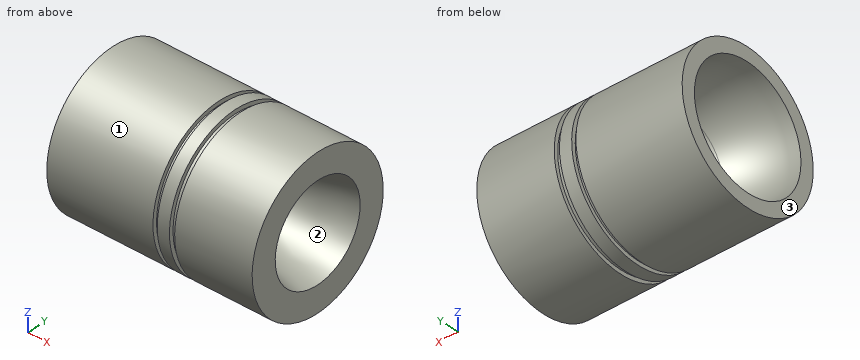
from build123d import *


with BuildPart() as part:
    # Sketch1 → Revolve1 (revolve)
    with BuildSketch(Plane.XY, mode=Mode.PRIVATE) as revolve1_sk:
        with BuildLine():
            Line((43.421005762, 29.901440031), (63.302799643, 18.422680981))
            ThreePointArc((63.302799643, 18.422680981), (68.543849717, 16.213738545), (74.168, 15.367))
            ThreePointArc((74.168, 15.367), (75.003256616, 15.406217174), (75.824358548, 15.564277983))
            Line((75.824358548, 15.564277983), (140.97, 33.02))
            Line((140.97, 33.02), (140.97, 50.927))
            Line((140.97, 50.927), (87.788503876, 50.927))
            Line((87.788503876, 50.927), (87.788503876, 48.180233369))
            Line((87.788503876, 48.180233369), (84.218492297, 48.180233369))
            Line((84.218492297, 48.180233369), (84.218492297, 50.927))
            Line((84.218492297, 50.927), (75.824358548, 50.927))
            Line((75.824358548, 50.927), (75.824358548, 48.180233369))
            Line((75.824358548, 48.180233369), (72.892938323, 48.180233369))
            Line((72.892938323, 48.180233369), (72.892938323, 50.927))
            Line((72.892938323, 50.927), (0, 50.927))
            Line((0, 50.927), (0, 41.402))
            ThreePointArc((0, 41.402), (22.475975666, 38.541805218), (43.421005762, 29.901440031))
        make_face()
    revolve(revolve1_sk.sketch.rotate(Axis((0, 0, 0), (1, 0, 0)), 90), axis=Axis((0, 0, 0), (1, 0, 0)))


solid = part.part
Work out the finished part from the listing and answer in its coordinate system (mm). Face numbers are marked on the shaded views. Round coordinates to 2 decimals unless told otherwise and drop trailing zeros. Order: outer loops, then holes, each group sorted by start corner. A loop starts at its lowest first (then second) coordinate and runs counter-clockwise, first axis right, second up. Notation, with made-up numbers: M 65.25,28 L 78.25,28 A13 cw 78.25,51 Z; hole C 22.5,80.5 d10. An arc over 180 degrees is marked long. Put each result on its own line as item: value. Start each with the question number.
Q1. Flat-ended cylindrical pins translate along their axes: pin 1 (6 mm diameter, centred on y = -16.5, z = -13, fed in from -X); pin 2 (1 mm diameter, centred on x = 121, y = -37.5, fed in from +Z); pin 3 (8 mm diameter, centred on x = 95.5, y = -27, fed in from -Z). Find the tip coordinate at first contact, or state that the pin passes through.
Q2. Section A-A, the plane x = 57 is taken. Write down the section's boundary in (y, z).
Q3. For a pull along Y with two mould halves and no side action, classify the marked faces 1, 2 and 3 as pulls with the +Y half, pulls with the -Y half, needs draft (parallel to the pull), parting line crosses it, or undercut.
Q4. Straight lines are drawn through the part: L1, parallel to Y at x = 25.5, z = -5; L2, parallel to Y at x = 18, z = -34.5; L3, parallel to Z at x = 71.5, y = 13. For each, find the intervals that lie inside material, in ascending order. Write a range as [from, to].
Findings below:
1. pin 1: stops at x = 53.63
1. pin 2: stops at z = 34.99
1. pin 3: stops at z = -45.44
2. outline: C 0,0 d101.85; hole C 0,0 d44.12
3. face 1: parting line crosses it
3. face 2: undercut
3. face 3: needs draft
4. L1: y = [-50.68, -37.35], [37.35, 50.68]
4. L2: y = [-37.46, -19.44], [19.44, 37.46]
4. L3: z = [-49.24, -8.6], [8.6, 49.24]
